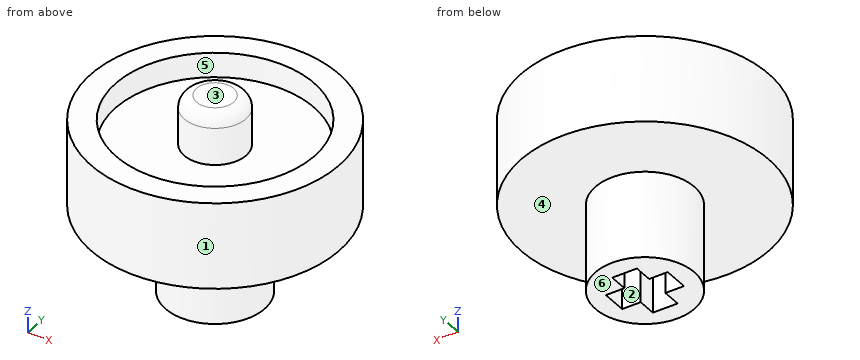
Autodesk Inventor part; units mm, degrees
ref_plane "YZ Plane" through (0, 0, 0) normal (1, 0, 0) x (0, 1, 0)
ref_plane "XZ Plane" through (0, 0, 0) normal (0, 1, 0) x (-1, 0, 0)
ref_plane "XY Plane" through (0, 0, 0) normal (0, 0, 1) x (1, 0, 0)
sketch "Sketch1" plane through (0, 0, 0) normal (0, 0, 1) x (1, 0, 0)
  circle A0 centre (0, 0) radius 10
  dimension "d0" = 20
extrude "Extrusion1" add sketch "Sketch1" along normal blind 5
sketch "Sketch2" plane through (0, 0, 0) normal (0, 0, -1) x (-1, 0, 0)
  circle A0 centre (0, 0) radius 4
  dimension "d3" = 8
extrude "Extrusion2" add sketch "Sketch2" along normal blind 7
sketch "Sketch3" plane through (0, 0, 5) normal (0, 0, 1) x (1, 0, 0)
  circle A0 centre (0, 0) radius 2.5
  dimension "d6" = 5
extrude "Extrusion3" add sketch "Sketch3" along normal blind 4
fillet "Fillet1" radius 1 1 edges at (-2.5, 0, 9)
sketch "Sketch4" plane through (0, 0, 5) normal (0, 0, 1) x (1, 0, 0)
  circle A0 centre (0, 0) radius 8
  circle A1 centre (0, 0) radius 10
  dimension "d10" = 2
  dimension "d11" = 20
extrude "Extrusion4" add sketch "Sketch4" along normal blind 2
sketch "Sketch5" plane through (0, 0, -7) normal (0, 0, -1) x (-1, 0, 0)
  line L0 (2.5, 1) -> (2.5, -1)
  line L1 (-2.5, -1) -> (-2.5, 1)
  line L2 (-1, 2.5) -> (1, 2.5)
  line L3 (1, -2.5) -> (-1, -2.5)
  line L4 (-2.5, 1) -> (-1, 1)
  line L5 (1, 1) -> (2.5, 1)
  line L6 (-1, -2.5) -> (-1, -1)
  line L7 (-1, 1) -> (-1, 2.5)
  line L8 (2.5, -1) -> (1, -1)
  line L9 (-1, -1) -> (-2.5, -1)
  line L10 (1, 2.5) -> (1, 1)
  line L11 (1, -1) -> (1, -2.5)
  point P0 (0, 0)
  dimension "d14" = 5
  dimension "d15" = 5
  dimension "d16" = 2
  dimension "d17" = 2
  dimension "d20" = 2.5
  dimension "d21" = 2.5
extrude "Extrusion5" cut sketch "Sketch5" against normal blind 10
properties part number "ArmClutchInsert"
Check sheet for the modelled part. Datum: model origin and axes. Units: mm. Face numbers are marked on the shaded views. A direction names the side the tool comes from. Give positions to 0.01 mm unless a question says otherwise; leave off trailing zeros. Loops run counter-clockwise (first coordinate to the right, second up) from the corner with the lowest first, then second, coordinate; pieces in that order, holes last. Notation, with made-up numbers: M -12,23.5 L 40,23.5 A23 ccw 40,32.5 Z; hole C -21,75 d4. An arc over 180 degrees is marked long. Use a Markdown table: item, result. Add a question column.
Q1. Tool access check on the marked faces 4, 5 and 6. Record the directions out of +Z, -Z, +X, -X, +Y, -Y that give a thin tool (end or side, any length) a straight path to the whole face; none if there is none.
Q2. Scan lines: line 1 along Y through (x, z) = (0, 5.6); line 2 along Y through (x, z) = (6, 2.25); line 3 along Z through (x, y) = (0.25, -4.5). Record each from-to range of solid material in increasing order. Write a range as [from, to].
Q3. Sectioned sample at B-B, the plane y = -6. Record the cut outline in (x, z).
Q4. Go/stop test with flat-tipped pins: pin 1 (1 mm diameter, centred on x = -4, z = -3, fed in from -Y); pin 2 (1.2 mm diameter, centred on y = -1.5, z = -0.5, fed in from +X); pin 3 (2 mm diameter, centred on y = -2.5, z = 5, fed in from -X). Record where each tip stops, or that it passes through.
Q5. Sectioned sample at A-A, the plane z = -2. Record the cut outline in (x, y), then the cut area to 3 significant figures.
Q6. Mould release check, pull along X, two halves, no side actions. Record for the marked faces 1, 2 and 3: pulls with the +X half, pulls with the -X half, needs draft (parallel to the pull), parting line crosses it, or undercut.
Q7. Sectioned sample at C-C, the plane x = 0. Record the cut outline in (y, z), then the cut area to 3 significant figures.
Verdict:
| question | item | result |
|---|---|---|
| 1 | face 4 | -Z |
| 1 | face 5 | +Z |
| 1 | face 6 | -Z, +X, -X, +Y, -Y |
| 2 | line 1 | [-10, -8], [-2.5, 2.5], [8, 10] |
| 2 | line 2 | [-8, 8] |
| 2 | line 3 | [0, 5] |
| 3 | outline | M -8,0 L 8,0 L 8,7 L 5.29,7 L 5.29,5 L -5.29,5 L -5.29,7 L -8,7 Z |
| 4 | pin 1 | y = -1.94 |
| 4 | pin 2 | x = 9.93 |
| 4 | pin 3 | x = -9.89 |
| 5 | outline | C 0,0 d8; hole M -2.5,-1 L -1,-1 L -1,-2.5 L 1,-2.5 L 1,-1 L 2.5,-1 L 2.5,1 L 1,1 L 1,2.5 L -1,2.5 L -1,1 L -2.5,1 Z |
| 5 | area | 34.3 mm^2 |
| 6 | face 1 | parting line crosses it |
| 6 | face 2 | undercut |
| 6 | face 3 | needs draft |
| 7 | outline | M -10,0 L -4,0 L -4,-7 L -2.5,-7 L -2.5,3 L 2.5,3 L 2.5,-7 L 4,-7 L 4,0 L 10,0 L 10,7 L 8,7 L 8,5 L 2.5,5 L 2.5,8 A1 ccw 1.5,9 L -1.5,9 A1 ccw -2.5,8 L -2.5,5 L -8,5 L -8,7 L -10,7 Z |
| 7 | area | 134 mm^2 |
